from build123d import *

# Parameters (mm, degrees)
F0_W          = 10
F0_H          = 6
F2_DEPTH      = 50.001
F2_DEPTH_BACK = 50.001


with BuildPart() as f1:
    # F0 (on Top) → F1 (revolve)
    with BuildSketch(Plane.XY):
        with BuildLine():
            Line((-33.7744166376, 0), (-53.7744166376, 0))
            Line((-53.7744166376, 0), (-53.7744166376, -35))
            Line((-53.7744166376, -35), (-3.7744166376, -35))
            Line((-3.7744166376, -35), (-3.7744166376, -20))
            Line((-3.7744166376, -20), (-28.7744166376, -20))
            ThreePointArc((-28.7744166376, -20), (-32.3099505436, -18.5355339059), (-33.7744166376, -15))
            Line((-33.7744166376, -15), (-33.7744166376, 0))
        make_face()
    revolve(axis=Axis((-3.7744166376, -50, 0), (1, 0, 0)))

    # F0 (on Top) → F2 (cut, two sides)
    with BuildSketch(Plane.XY) as f2_sk:
        with Locations((-48.7744166376, -53)):
            Rectangle(F0_W, F0_H)
        with Locations((-48.7744166376, -47)):
            Rectangle(F0_W, F0_H)
    extrude(amount=-F2_DEPTH, mode=Mode.SUBTRACT)
    extrude(f2_sk.sketch, amount=F2_DEPTH_BACK, mode=Mode.SUBTRACT)


solid = f1.part
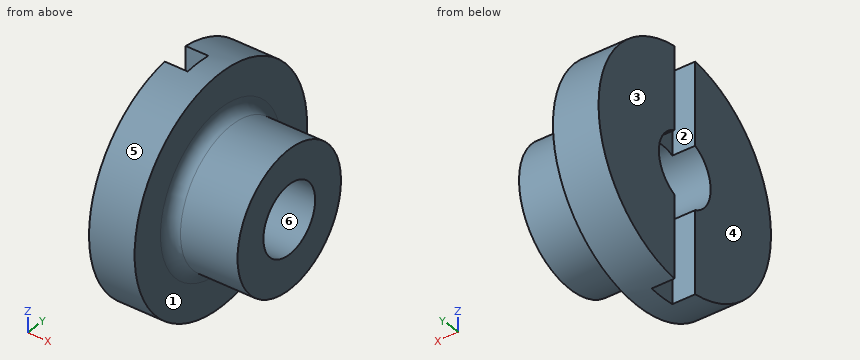
Can you work these out from the model? Positions are in its coordinate system, mm. Face numbers are marked on the shaded views. A direction names the side the tool comes from. Give positions to 0.01 mm unless a question says otherwise; leave off trailing zeros. Loops run counter-clockwise (first coordinate to the right, second up) from the corner with the lowest first, then second, coordinate; pieces in that order, holes last. Notation, with made-up numbers: (60.25, 31) -> (98.25, 31) arc R24 ccw to (98.25, 61) -> close; hole circle Ø1 at (-35, -30.75). An arc over 180 degrees is marked (long way). Use one line per item in the form item = value.
1) If we section it at C-C (z = 0): Please give me the cut outline in (x, y).
Answers:
outline = (-53.77, -100) -> (-33.77, -100) -> (-33.77, -85) arc R5 cw to (-28.77, -80) -> (-3.77, -80) -> (-3.77, -65) -> (-53.77, -65) -> close; (-53.77, -35) -> (-3.77, -35) -> (-3.77, -20) -> (-28.77, -20) arc R5 cw to (-33.77, -15) -> (-33.77, 0) -> (-53.77, 0) -> close
2) For the marked faces 1, 2 and 3, which set-ups out of +Z, -Z, +X, -X, +Y, -Y let a thin tool reach every point of the face, with its end or its side?
Answers:
face_1 = +X
face_2 = +Z, -Z, -X
face_3 = +Z, -Z, -X, +Y, -Y
3) I need wall thicknesses on line 1 along Z through (x, y) = (-19.5, -50); line 2 along Z through (x, y) = (-43, -50); line 3 along Y through (x, z) = (-38, 0). Which ranges of each line are inside material? Lowest first, please.
Answers:
line_1 = -30 to -15, 15 to 30
line_2 = -50 to -15, 15 to 50
line_3 = -100 to -65, -35 to 0
4) If we section it at D-D (x = -20): Please give me the cut outline in (y, z).
Answers:
outline = circle Ø60 at (-50, 0); hole circle Ø30 at (-50, 0)
5) If we section it at B-B (x = -47.5): Please give me the cut outline in (y, z).
Answers:
outline = (-56, -49.64) -> (-56, -13.75) arc R15 cw to (-56, 13.75) -> (-56, 49.64) arc R50 ccw to start; (-44, -49.64) arc R50 ccw to (-44, 49.64) -> (-44, 13.75) arc R15 cw to (-44, -13.75) -> close
6) Will these pins go through, and if not, where does the flat tip stop? pin 1 (1 mm diameter, centred on x = -9.5, y = -59.5, fed in from -Z); pin 2 (8 mm diameter, centred on x = -48.5, y = -12.5, fed in from -Z); pin 3 (11 mm diameter, centred on x = -47.5, z = 29, fed in from -Y).
Answers:
pin_1 = -28.62
pin_2 = -37.12
pin_3 = -94.13
7) We'd pull the mould along Y, two halves only. Please class the marked faces 4, 5 and 6: released by +Y, released by -Y, zero draft, split by the parting line, or undercut.
Answers:
face_4 = zero draft
face_5 = split by the parting line
face_6 = undercut
8) If we section it at A-A (y = -50): Please give me the cut outline in (x, z), plus the area to 3 significant figures.
Answers:
outline = (-43.77, -50) -> (-33.77, -50) -> (-33.77, -35) arc R5 cw to (-28.77, -30) -> (-3.77, -30) -> (-3.77, -15) -> (-43.77, -15) -> close; (-43.77, 15) -> (-3.77, 15) -> (-3.77, 30) -> (-28.77, 30) arc R5 cw to (-33.77, 35) -> (-33.77, 50) -> (-43.77, 50) -> close
area = 1,610 mm²
